from build123d import *

# Parameters (mm, degrees)
SKETCH_2_W          = 40
SKETCH_2_H          = 20
EXTRUDE_1_DEPTH     = 485
SKETCH_3_R          = 4.75
CUT_EXTRUDE_1_DEPTH = 486
SKETCH_4_W          = 4.2
SKETCH_4_H          = 485
CUT_EXTRUDE_2_DEPTH = 3
SKETCH_5_W          = 4.2
SKETCH_5_H          = 485
CUT_EXTRUDE_3_DEPTH = 4


with BuildPart() as part:
    # 草图2 → 凸台-拉伸1 (new body)
    with BuildSketch(Plane(origin=(0, 0, 0), x_dir=(1, 0, 0), z_dir=(0, 1, 0))):
        Rectangle(SKETCH_2_W, SKETCH_2_H)
    extrude(amount=EXTRUDE_1_DEPTH)

    # 草图3 → 切除-拉伸1 (cut, through all)
    with BuildSketch(Plane.XZ):
        with Locations((-10, 0)):
            Circle(SKETCH_3_R)
        with Locations((10, 0)):
            Circle(SKETCH_3_R)
    extrude(amount=-CUT_EXTRUDE_1_DEPTH, mode=Mode.SUBTRACT)

    # 草图4 → 切除-拉伸2 (cut)
    with BuildSketch(Plane.XY.offset(10)):
        with Locations((-10.1, 242.5)):
            Rectangle(SKETCH_4_W, SKETCH_4_H)
        with Locations((10.1, 242.5)):
            Rectangle(SKETCH_4_W, SKETCH_4_H)
    extrude(amount=-CUT_EXTRUDE_2_DEPTH, mode=Mode.SUBTRACT)

    # 草图5 → 切除-拉伸3 (cut)
    with BuildSketch(Plane(origin=(0, 0, -10), x_dir=(-1, 0, 0), z_dir=(0, 0, -1))):
        with Locations((-10.1, 242.5)):
            Rectangle(SKETCH_5_W, SKETCH_5_H)
        with Locations((10.1, 242.5)):
            Rectangle(SKETCH_5_W, SKETCH_5_H)
    extrude(amount=-CUT_EXTRUDE_3_DEPTH, mode=Mode.SUBTRACT)


solid = part.part
Model file for the job. Use its own axes, mm. Give positions to 0.01 mm unless a question says otherwise; leave off trailing zeros. Order: outer loops, then holes, each group sorted by start corner. A loop starts at its lowest first (then second) coordinate and runs counter-clockwise, first axis right, second up. Notation, with made-up numbers: M -16.5,26.25 L -12.5,26.25 A13 ccw -12.5,37.25 Z; hole C -23.75,75 d2. An arc over 180 degrees is marked long. Put each result on its own line as item: value. Start each with the question number.
(1) Drill centre lines: L1, parallel to X at y = 39, z = 8.75; L2, parallel to Z at x = 10, y = 148.5; L3, parallel to X at y = 459.5, z = -2.25. Where is each one in solid material? Low to high. Write a range as [from, to].
(2) Pull direction X, two halves, no side cores. Call faces 1 (the face through (20, 239, 0)), 2 (the face through (8.97, 239.105, -4.637)), 3 (the face through (16, 239, 10)): released by +X, released by -X, zero draft, split by the parting line, or undercut.
(3) Pin check, flat tips, straight feed: pin 1 Ø2 at (x, y) = (-10.5, 198) entering from +Z; pin 2 Ø8.5 at (x, z) = (10, 0) entering from +Y. Stop position of each tip, or through.
(4) Band-saw the part on A-A on z = 0. Give the cut face in (x, y), then the cut area to 3 significant figures.
(5) Band-saw the part on B-B on y = 94. Give the cut face in (x, z).
Results below:
1. L1: x = [-20, -12.2], [-8, 8], [12.2, 20]
1. L2: z = [-6, -4.75], [4.75, 7]
1. L3: x = [-20, -14.18], [-5.82, 5.82], [14.18, 20]
2. face 1: released by +X
2. face 2: undercut
2. face 3: zero draft
3. pin 1: stops at z = 7
3. pin 2: passes through
4. outline: M -20,0 L -14.75,0 L -14.75,485 L -20,485 Z; M -5.25,0 L 5.25,0 L 5.25,485 L -5.25,485 Z; M 14.75,0 L 20,0 L 20,485 L 14.75,485 Z
4. area: 10,200 mm2
5. outline: M -20,-10 L -12.2,-10 L -12.2,-6 L -8,-6 L -8,-10 L 8,-10 L 8,-6 L 12.2,-6 L 12.2,-10 L 20,-10 L 20,10 L 12.2,10 L 12.2,7 L 8,7 L 8,10 L -8,10 L -8,7 L -12.2,7 L -12.2,10 L -20,10 Z; hole C -10,0 d9.5; hole C 10,0 d9.5
